Build history of the part. All positions in model axes, mm. Face numbers are marked on the shaded views. A direction names the side the tool comes from. Round coordinates to 2 decimals unless told otherwise and drop trailing zeros. Order: outer loops, then holes, each group sorted by start corner. A loop starts at its lowest first (then second) coordinate and runs counter-clockwise, first axis right, second up. Notation, with made-up numbers: M -20,6.5 L 4,6.5 A18 cw 4,40.5 Z; hole C 46.25,-29 d7. An arc over 180 degrees is marked long. One line per item, written item: value. Start each with the question number.
Item 1: Probe L1, parallel to X at y = -10, z = 14; L2, parallel to Z at x = -9.5, y = -15.5; L3, parallel to Y at x = 34.5, z = 23.5. List the from-to ranges inside material, lowest first.
Item 2: Pin check, flat tips, straight feed: pin 1 (12 mm diameter, centred on x = 57, y = 0.5, fed in from +Z); pin 2 (5 mm diameter, centred on y = 29, z = 31.5, fed in from +X); pin 3 (2 mm diameter, centred on x = -21, y = -25, fed in from +Z). Stop position of each tip, or through.
Item 3: Band-saw the part on A-A, the plane x = 60. Write the cut outline in (y, z), then the cut area to 3 significant figures.
Item 4: Band-saw the part on C-C, the plane x = -16.5. Write the cut outline in (y, z), then the cut area to 3 significant figures.
Item 5: Band-saw the part on B-B, the plane y = -1.5. Write the cut outline in (x, z).
Item 6: Tool access for the marked faces 1 and 2: list every direction of +Z, -Z, +X, -X, +Y, -Y with a clear straight run to the whole face (end or side of a thin tool).
Item 7: Band-saw the part on D-D, the plane z = 20. Write the cut outline in (x, y).
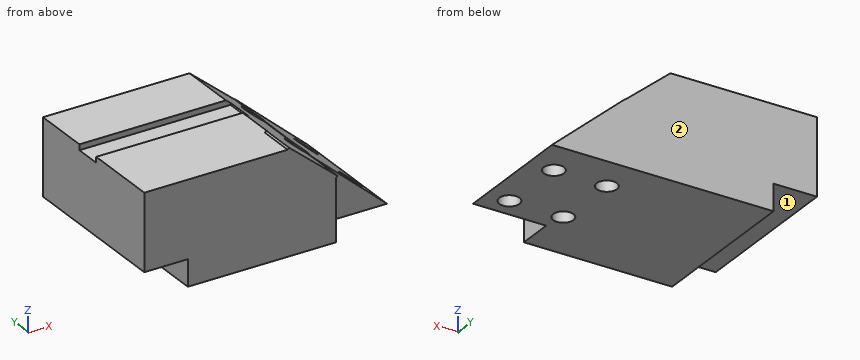
```python
from build123d import *

# Parameters (mm, degrees)
F0_R      = 5.0203932543
F0_W      = 36.212477833
F0_H      = 17.3722021282
F1_DEPTH  = 50.8
F2_W      = 36.2125001848
F2_H      = 17.3722039908
F3_DEPTH  = 50.8
F5_DEPTH  = 50.8
F7_DEPTH  = 50.8
F8_DEPTH  = 68.58
F9_DEPTH  = 1.016
F11_DEPTH = 63.5
F12_W     = 21.5317420661
F12_H     = 13.0903217942
F13_DEPTH = 76.2
F14_DEPTH = 25.4
F15_W     = 72.532140549
F15_H     = 13.0903217942
F16_DEPTH = 12.7
F17_W     = 4.0916903161
F17_H     = 13.0903217942
F18_DEPTH = 12.7
F19_DEPTH = 6.35
F20_DEPTH = 5.08
F21_DEPTH = 2.2606
F22_DEPTH = 2.032
F23_DEPTH = 1.524
F24_DEPTH = 1.016


with BuildPart() as f1:
    # F0 (on Top) → F1 (new body)
    with BuildSketch(Plane.XY):
        Polygon((-59.0899549425, 41.4730757475), (-59.0899549425, -37.5582128763), (35.8454622328, -37.5582128763), (35.8454622328, -20.1860107481), (72.0579400659, -20.1860107481), (72.0579400659, 41.4730757475), align=None)
        with Locations((33.8835379278, -9.9094957113)):
            Circle(F0_R, mode=Mode.SUBTRACT)
        with Locations((60.5580285192, -9.9094957113)):
            Circle(F0_R, mode=Mode.SUBTRACT)
        with Locations((33.153988421, 22.8774771094)):
            Circle(F0_R, mode=Mode.SUBTRACT)
        with Locations((59.3529156527, 22.8774771094)):
            Circle(F0_R, mode=Mode.SUBTRACT)
        with Locations((53.9517011493, -28.8721118122)):
            Rectangle(F0_W, F0_H)
    extrude(amount=F1_DEPTH)

    # F2 (on face) → F3 (cut)
    with BuildSketch(Plane.XY.offset(50.8)):
        with Locations((53.9516899735, -28.8721108809)):
            Rectangle(F2_W, F2_H)
    extrude(amount=-F3_DEPTH, mode=Mode.SUBTRACT)

    # F4 (on face) → F5 (join)
    with BuildSketch(Plane.XZ.offset(37.5582128763)):
        Polygon((11.8669271469, 50.8), (35.8454398811, 30.5626192379), (35.8454398811, 50.8), align=None)
    extrude(amount=F5_DEPTH)

    # F6 (on face) → F7 (cut)
    with BuildSketch(Plane.XY):
        Polygon((-59.0899549425, 40.9865353048), (-60.1052679121, 25.7568676025), (-59.0899549425, 25.7568676025), align=None)
        Polygon((-59.0484701097, 41.6088066995), (-59.0575188558, 41.4730757475), (-25.7593989372, 41.4730757475), (-25.7593989372, 41.6088066995), align=None)
        Polygon((-59.0899549425, 40.9865353048), (-59.0899549425, 25.7568676025), (-25.7593989372, 25.7568676025), (-25.7593989372, 41.4730757475), (-59.0575188558, 41.4730757475), align=None)
    extrude(amount=-F7_DEPTH, mode=Mode.SUBTRACT)

    # F8 (cut): a face of the model
    f8_faces = [f1.faces().sort_by_distance(p)[0] for p in [
        (27.852602303, -88.3582128763, 44.0542064126),
    ]]
    extrude(f8_faces, amount=-F8_DEPTH, mode=Mode.SUBTRACT)

    # F9 (add): a face of the model
    f9_faces = [f1.faces().sort_by_distance(p)[0] for p in [
        (23.856183514, -28.6682128763, 40.681309619),
    ]]
    extrude(f9_faces, amount=F9_DEPTH)

    # F8_face1 (on face) + F10 (on face) → F11 (cut)
    with BuildSketch(Plane(origin=(28.3776884562, -19.7782128763, 44.4973685275), x_dir=(1, 0, 0), z_dir=(0, -1, 0))):
        Polygon((7.4677514249, -12.6052629449), (7.4677514249, 6.3026314725), (-14.9355028497, 6.3026314725), align=None)
    with BuildSketch(Plane.XZ.offset(20.1860088855)):
        Polygon((35.8454398811, 32.1115117159), (72.0579400659, 0), (72.0579400659, 50.8), (35.8454398811, 50.8), align=None)
    extrude(amount=-F11_DEPTH, mode=Mode.SUBTRACT)

    # F12 (on face) → F13 (cut)
    with BuildSketch(Plane.XZ.offset(37.5582128763)):
        with Locations((-48.3240839094, 6.5451608971)):
            Rectangle(F12_W, F12_H)
    extrude(amount=-F13_DEPTH, mode=Mode.SUBTRACT)

    # F14 (cut): a face of the model
    f14_faces = [f1.faces().sort_by_distance(p)[0] for p in [
        (-48.3240839094, 38.6417871237, 6.5451608971),
    ]]
    extrude(f14_faces, amount=-F14_DEPTH, mode=Mode.SUBTRACT)

    # F15 (on face) → F16 (cut)
    with BuildSketch(Plane.XY.offset(50.8)):
        with Locations((-22.823884668, 6.5451608971)):
            Rectangle(F15_W, F15_H)
    extrude(amount=-F16_DEPTH, mode=Mode.SUBTRACT)

    # F17 (on face) → F18 (cut)
    with BuildSketch(Plane(origin=(30.6307366038, 0, 36.2932098944), x_dir=(0.7642049157, 0, -0.6449735241), z_dir=(0.6449735241, 0, 0.7642049157))):
        with Locations((-20.446225546, 6.5451608971)):
            Rectangle(F17_W, F17_H)
    extrude(amount=-F18_DEPTH, mode=Mode.SUBTRACT)

    # F19 (add): a face of the model
    f19_faces = [f1.faces().sort_by_distance(p)[0] for p in [
        (-22.823884668, 6.5451608971, 38.1),
    ]]
    extrude(f19_faces, amount=F19_DEPTH)

    # F20 (add): a face of the model
    f20_faces = [f1.faces().sort_by_distance(p)[0] for p in [
        (-22.823884668, 6.5451608971, 44.45),
    ]]
    extrude(f20_faces, amount=F20_DEPTH)

    # F21 (add): a face of the model
    f21_faces = [f1.faces().sort_by_distance(p)[0] for p in [
        (13.4421856065, 6.5451608971, 46.9930168384),
    ]]
    extrude(f21_faces, amount=F21_DEPTH)

    # F22 (cut): a face of the model
    f22_faces = [f1.faces().sort_by_distance(p)[0] for p in [
        (-21.693584668, 6.5451608971, 49.53),
    ]]
    extrude(f22_faces, amount=-F22_DEPTH, mode=Mode.SUBTRACT)

    # F23 (add): a face of the model
    f23_faces = [f1.faces().sort_by_distance(p)[0] for p in [
        (-21.693584668, 6.5451608971, 47.498),
    ]]
    extrude(f23_faces, amount=F23_DEPTH)

    # F24 (cut): a face of the model
    f24_faces = [f1.faces().sort_by_distance(p)[0] for p in [
        (-21.693584668, 6.5451608971, 49.022),
    ]]
    extrude(f24_faces, amount=-F24_DEPTH, mode=Mode.SUBTRACT)


solid = f1.part
```
Output:
1. L1: x = -59.09 to 28.86, 38.9 to 55.54
1. L2: z = 0 to 50.8
1. L3: y = -37.56 to -14.89, -4.93 to 18.04, 27.71 to 41.47
2. pin 1: stops at z = 18.67
2. pin 2: stops at x = 39.35
2. pin 3: stops at z = 50.8
3. outline: M -20.19,0 L -14.9,0 L -14.9,10.69 L -20.19,10.69 Z; M -4.92,0 L 17.9,0 L 17.9,10.69 L -4.92,10.69 Z; M 27.86,0 L 41.47,0 L 41.47,10.69 L 27.86,10.69 Z
3. area: 446 mm²
4. outline: M -37.56,0 L 41.47,0 L 41.47,50.8 L 13.09,50.8 L 13.09,48.01 L 0,48.01 L 0,50.8 L -37.56,50.8 Z
4. area: 3,980 mm²
5. outline: M -59.09,13.09 L -37.56,13.09 L -37.56,0 L 72.06,0 L 35.85,32.11 L 35.85,31.89 L 13.44,50.8 L -59.09,50.8 Z
6. face 1: -Z, -X, +Y, -Y
6. face 2: +Z, -Z, +X, -X, +Y
7. outline: M -59.09,-37.56 L 35.85,-37.56 L 35.85,-20.19 L 49.5,-20.19 L 49.5,41.47 L -59.09,41.47 Z; hole C 33.15,22.88 d10.04; hole C 33.88,-9.91 d10.04
